from build123d import *

# Parameters (mm, degrees)
SKETCH1_R           = 1.5
SKETCH1_W           = 55
SKETCH1_H           = 55
BOSS_EXTRUDE1_DEPTH = 3
FILLET1_R           = 10


with BuildPart() as part:
    # Sketch1 → Boss-Extrude1 (new body)
    with BuildSketch(Plane(origin=(0, 0, 0), x_dir=(1, 0, 0), z_dir=(0, 1, 0))):
        Polygon((-60, 130), (60, 130), (60, 35), (111, 35), (111, -35), (-111, -35), (-111, 35), (-60, 35), align=None)
        with Locations(Location((38, 118.5, 0), (0, 0, 270))):
            Circle(SKETCH1_R, mode=Mode.SUBTRACT)
        with Locations(Location((38, 46.5, 0), (0, 0, 270))):
            Circle(SKETCH1_R, mode=Mode.SUBTRACT)
        with Locations(Location((-38, 118.5, 0), (0, 0, 270))):
            Circle(SKETCH1_R, mode=Mode.SUBTRACT)
        with Locations(Location((-38, 46.5, 0), (0, 0, 270))):
            Circle(SKETCH1_R, mode=Mode.SUBTRACT)
        with Locations(Location((-15, 6.5, 0), (0, 0, 270))):
            Circle(SKETCH1_R, mode=Mode.SUBTRACT)
        with Locations(Location((15, 6.5, 0), (0, 0, 270))):
            Circle(SKETCH1_R, mode=Mode.SUBTRACT)
        with Locations(Location((15, -23.5, 0), (0, 0, 270))):
            Circle(SKETCH1_R, mode=Mode.SUBTRACT)
        with Locations(Location((-15, -23.5, 0), (0, 0, 270))):
            Circle(SKETCH1_R, mode=Mode.SUBTRACT)
        with Locations(Location((-50, 82.5, 0), (0, 0, 270))):
            Circle(SKETCH1_R, mode=Mode.SUBTRACT)
        with Locations(Location((-101, 25, 0), (0, 0, 270))):
            Circle(SKETCH1_R, mode=Mode.SUBTRACT)
        with Locations(Location((-101, -25, 0), (0, 0, 90))):
            Circle(SKETCH1_R, mode=Mode.SUBTRACT)
        with Locations(Location((-31, 25, 0), (0, 0, 270))):
            Circle(SKETCH1_R, mode=Mode.SUBTRACT)
        with Locations(Location((-31, -25, 0), (0, 0, 90))):
            Circle(SKETCH1_R, mode=Mode.SUBTRACT)
        with Locations(Location((101, 25, 0), (0, 0, 90))):
            Circle(SKETCH1_R, mode=Mode.SUBTRACT)
        with Locations(Location((101, -25, 0), (0, 0, 270))):
            Circle(SKETCH1_R, mode=Mode.SUBTRACT)
        with Locations(Location((31, -25, 0), (0, 0, 270))):
            Circle(SKETCH1_R, mode=Mode.SUBTRACT)
        with Locations(Location((31, 25, 0), (0, 0, 90))):
            Circle(SKETCH1_R, mode=Mode.SUBTRACT)
        with Locations(Location((50, 82.5, 0), (0, 0, 90))):
            Circle(SKETCH1_R, mode=Mode.SUBTRACT)
        with BuildLine():
            Line((74.5, -16.5), (67.5, -16.5))
            ThreePointArc((67.5, -16.5), (66, -15), (67.5, -13.5))
            Line((67.5, -13.5), (74.5, -13.5))
            ThreePointArc((74.5, -13.5), (76, -15), (74.5, -16.5))
        make_face(mode=Mode.SUBTRACT)
        with BuildLine():
            Line((74.5, 13.5), (67.5, 13.5))
            ThreePointArc((67.5, 13.5), (66, 15), (67.5, 16.5))
            Line((67.5, 16.5), (74.5, 16.5))
            ThreePointArc((74.5, 16.5), (76, 15), (74.5, 13.5))
        make_face(mode=Mode.SUBTRACT)
        with BuildLine():
            Line((92.5, 16.5), (99.5, 16.5))
            ThreePointArc((99.5, 16.5), (101, 15), (99.5, 13.5))
            Line((99.5, 13.5), (92.5, 13.5))
            ThreePointArc((92.5, 13.5), (91, 15), (92.5, 16.5))
        make_face(mode=Mode.SUBTRACT)
        with BuildLine():
            Line((92.5, -13.5), (99.5, -13.5))
            ThreePointArc((99.5, -13.5), (101, -15), (99.5, -16.5))
            Line((99.5, -16.5), (92.5, -16.5))
            ThreePointArc((92.5, -16.5), (91, -15), (92.5, -13.5))
        make_face(mode=Mode.SUBTRACT)
        with BuildLine():
            Line((-92.5, -16.5), (-99.5, -16.5))
            ThreePointArc((-99.5, -16.5), (-101, -15), (-99.5, -13.5))
            Line((-99.5, -13.5), (-92.5, -13.5))
            ThreePointArc((-92.5, -13.5), (-91, -15), (-92.5, -16.5))
        make_face(mode=Mode.SUBTRACT)
        with BuildLine():
            Line((-92.5, 13.5), (-99.5, 13.5))
            ThreePointArc((-99.5, 13.5), (-101, 15), (-99.5, 16.5))
            Line((-99.5, 16.5), (-92.5, 16.5))
            ThreePointArc((-92.5, 16.5), (-91, 15), (-92.5, 13.5))
        make_face(mode=Mode.SUBTRACT)
        with BuildLine():
            Line((-74.5, -13.5), (-67.5, -13.5))
            ThreePointArc((-67.5, -13.5), (-66, -15), (-67.5, -16.5))
            Line((-67.5, -16.5), (-74.5, -16.5))
            ThreePointArc((-74.5, -16.5), (-76, -15), (-74.5, -13.5))
        make_face(mode=Mode.SUBTRACT)
        with BuildLine():
            Line((-74.5, 16.5), (-67.5, 16.5))
            ThreePointArc((-67.5, 16.5), (-66, 15), (-67.5, 13.5))
            Line((-67.5, 13.5), (-74.5, 13.5))
            ThreePointArc((-74.5, 13.5), (-76, 15), (-74.5, 16.5))
        make_face(mode=Mode.SUBTRACT)
        with Locations((0, 82.5)):
            Rectangle(SKETCH1_W, SKETCH1_H, mode=Mode.SUBTRACT)
    extrude(amount=BOSS_EXTRUDE1_DEPTH)

    # Fillet1
    fillet1_edges = [part.edges().sort_by_distance(p)[0] for p in [
        (111, 1.5, -35),
        (111, 1.5, 35),
        (-111, 1.5, 35),
        (-111, 1.5, -35),
        (-60, 1.5, -130),
        (60, 1.5, -130),
    ]]
    fillet(fillet1_edges, radius=FILLET1_R)


solid = part.part
Geometry: final body of the model. Coordinates: model frame, mm. Coordinates: 2 decimals unless noted, no trailing zeros. Order: outer loops, then holes, each group sorted by start corner. A loop starts at its lowest first (then second) coordinate and runs counter-clockwise, first axis right, second up.
1) Section A-A (z = -100.5). Return loops of the section in (x, y), then the cut area to 3 significant figures.
Result sheet:
outline: (-60, 0) - (-27.5, 0) - (-27.5, 3) - (-60, 3) - close; (27.5, 0) - (60, 0) - (60, 3) - (27.5, 3) - close
area: 195 mm2
2) First-contact query: P1, Ø0.9, axis at x = -78.5, y = 2, coming from the -Z side; P2, Ø1.5, axis at y = 1.5, z = -95, coming from the +X side; P3, Ø1.8, axis at x = -15, z = 23.5, coming from the -Y side. Flat tips, straight axial feed; report the tip coordinate or a pass-through.
Result sheet:
P1: stops at z = -35
P2: stops at x = 60
P3: passes through
3) Section B-B (x = 0). Return loops of the section in (y, z).
Result sheet:
outline: (0, -130) - (3, -130) - (3, -110) - (0, -110) - close; (0, -55) - (3, -55) - (3, 35) - (0, 35) - close
4) Ray query, probe 1 along X at (y, z) = (0.75, -25); probe 2 along X at (y, z) = (1.2, -108); probe 3 along Z at (x, y) = (-74, 2.3). Return the intervals inside material, ascending.
Result sheet:
probe 1: x = -111 to -102.5, -99.5 to -32.5, -29.5 to 29.5, 32.5 to 99.5, 102.5 to 111
probe 2: x = -60 to -27.5, 27.5 to 60
probe 3: z = -35 to -16.5, -13.5 to 13.5, 16.5 to 35
5) Section C-C (y = 1.6). Give the number of separate pieces and of enclosed holes in the cut face, then the cut area to 3 significant figures.
Result sheet:
separate pieces: 1
enclosed holes: 27
area: 23,400 mm2
